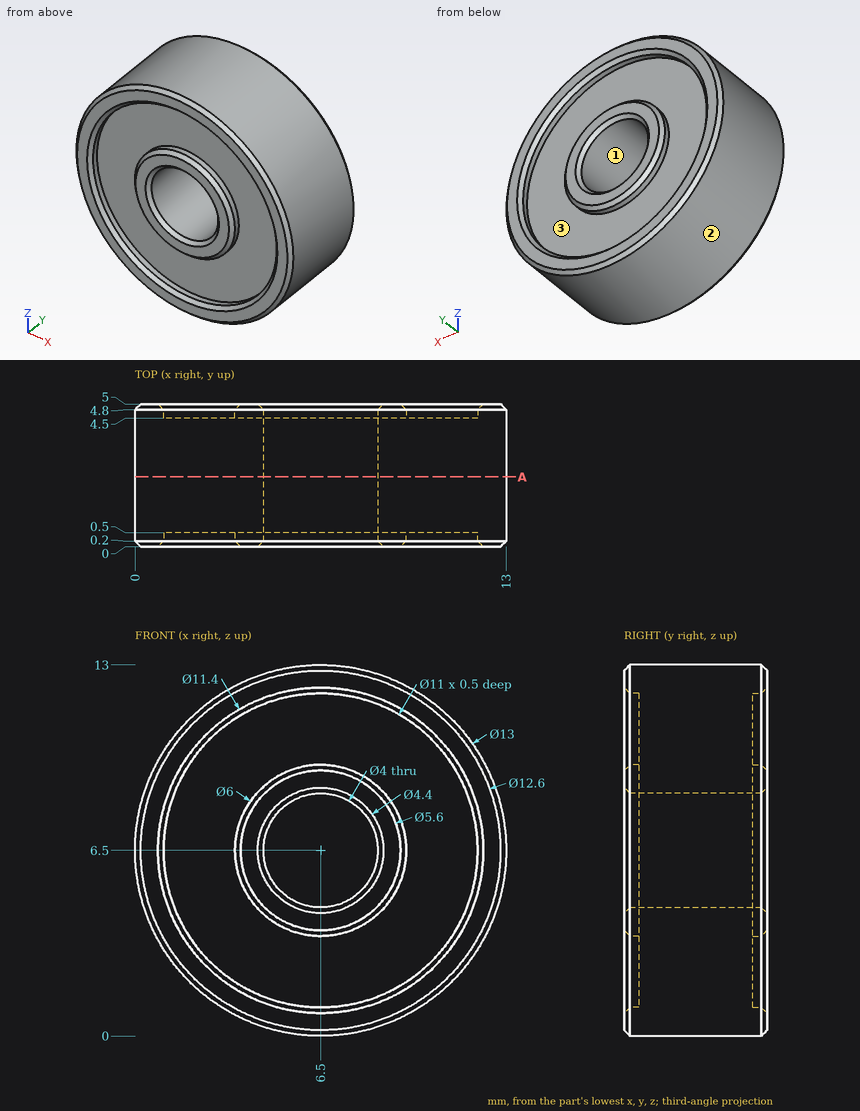
Study the drawing (mm; zero at the part's minimum x, y, z) and answer. Give positions to 0.01 mm unless a question says otherwise; leave off trailing zeros. Order: outer loops, then holes, each group sorted by start corner. A loop starts at its lowest first (then second) coordinate and runs counter-clockwise, first axis right, second up. Notation, with made-up numbers: (42, 34.25) - (57, 34.25) arc R21 cw to (57, 61.25) - close; hole circle Ø10 at (2.5, -38.75). An arc over 180 degrees is marked (long way). Use one line per item in the form item = value. Start each with the question number.
(1) A cutting plane is placed at A-A, the plane y = 2.45. Write down the section's boundary in (x, z), then the cut area to 3 significant figures.
(2) Flat-ended cylindrical pins translate along their axes: pin 1 Ø5 at (x, z) = (4, 2.5) entering from -Y; pin 2 Ø1.5 at (x, z) = (7, 7) entering from +Y; pin 3 Ø1.5 at (y, z) = (2.5, 9) entering from -X; pin 4 Ø2 at (x, y) = (9, 2.5) entering from +Z. Find the tip coordinate at first contact, or state that the pin passes through.
(3) The mould has two halves that part along X. Classify the marked faces 1, 2 and 3: released by +X, released by -X, zero draft, split by the parting line, or undercut.
(4) Consider line 1 (Z direction, x = 6.5, y = 0.3); line 2 (Z direction, x = 6.5, y = 2.7); line 3 (Y direction, x = 5.5, z = 3.25). Determine where each line is inside the solid, lowest interval first. Write a range as from..to.
Ans:
q1.outline = circle Ø13 at (6.5, 6.5); hole circle Ø4 at (6.5, 6.5)
q1.area = 120 mm^2
q2.pin_1 = 0
q2.pin_2 = through
q2.pin_3 = 0.24
q2.pin_4 = 12.82
q3.face_1 = undercut
q3.face_2 = split by the parting line
q3.face_3 = undercut
q4.line_1 = 0..1, 3.5..4.5, 8.5..9.5, 12..13
q4.line_2 = 0..4.5, 8.5..13
q4.line_3 = 0.5..4.5
